The listing builds one solid part. Answer for the finished solid, in the listing's coordinates (mm). A direction names the side the tool comes from. Give positions to 0.01 mm unless a question says otherwise; leave off trailing zeros. Write each loop counter-clockwise with the first axis right and the second up, starting at its lowest first coordinate (ties: lowest second). Pieces come first, ordered by that corner, then holes. Notation, with made-up numbers: M 52.25,38 L 75.25,38 A18 cw 75.25,71 Z; hole C 12,-22.5 d9. An arc over 180 degrees is marked long. Answer as a JSON object with one key per item and string values.
```python
from build123d import *

# Parameters (mm, degrees)
SKETCH1_W               = 381
SKETCH1_H               = 76.2
BOSS_EXTRUDE1_DEPTH     = 14
SKETCH2_W               = 353.0000052
SKETCH2_H               = 48.2
CUT_EXTRUDE1_DEPTH      = 14
SKETCH5_W               = 381
SKETCH5_H               = 13.97
BOSS_EXTRUDE2_DEPTH     = 76.2
SKETCH6_W               = 353.0000052
SKETCH6_H               = 48.2
CUT_EXTRUDE2_DEPTH      = 76.2
SKETCH3_W               = 13.9999974
SKETCH3_H               = 14
BOSS_EXTRUDE3_DEPTH     = 429.26
SKETCH7_W               = 13.9999974
SKETCH7_H               = 101.6
CUT_EXTRUDE3_DEPTH      = 429.26
SKETCH10_W              = 13.9999974
SKETCH10_H              = 13.97
BOSS_EXTRUDE4_DEPTH     = 48.26
SKETCH11_W              = 353.0000052
SKETCH11_H              = 13.97
BOSS_EXTRUDE5_DEPTH     = 76.2
CUT_EXTRUDE4_DEPTH      = 352.863349754
CUT_EXTRUDE4_DEPTH_BACK = 352.863349754
SKETCH12_W              = 353.0000052
SKETCH12_H              = 48.2
SKETCH13_W              = 13.97
SKETCH13_H              = 13.97
BOSS_EXTRUDE6_DEPTH     = 48.26


with BuildPart() as part:
    # Sketch1 → Boss-Extrude1 (new body)
    with BuildSketch(Plane.XY):
        Rectangle(SKETCH1_W, SKETCH1_H)
    extrude(amount=BOSS_EXTRUDE1_DEPTH)

    # Sketch2 → Cut-Extrude1 (cut)
    with BuildSketch(Plane.XY.offset(14)):
        Rectangle(SKETCH2_W, SKETCH2_H)
    extrude(amount=-CUT_EXTRUDE1_DEPTH, mode=Mode.SUBTRACT)



with BuildPart() as body_2:
    # Sketch5 → Boss-Extrude2 (new body)
    with BuildSketch(Plane(origin=(0, -38.1, 0), x_dir=(1, 0, 0), z_dir=(0, 1, 0))):
        with Locations((0, -450.215)):
            Rectangle(SKETCH5_W, SKETCH5_H)
    extrude(amount=BOSS_EXTRUDE2_DEPTH)

    # Sketch6 → Cut-Extrude2 (cut)
    with BuildSketch(Plane(origin=(0, 0, 443.23), x_dir=(-1, 0, 0), z_dir=(0, 0, -1))):
        Rectangle(SKETCH6_W, SKETCH6_H)
    extrude(amount=-CUT_EXTRUDE2_DEPTH, mode=Mode.SUBTRACT)


with BuildPart() as part_1:
    add(part.part)

    add(body_2.part)  # Boss-Extrude3 merges body 2
    # Sketch3 → Boss-Extrude3 (add)
    with BuildSketch(Plane.XY.offset(14)):
        with Locations((-183.5000013, -31.1)):
            Rectangle(SKETCH3_W, SKETCH3_H)
        with Locations((-183.5000013, 31.1)):
            Rectangle(SKETCH3_W, SKETCH3_H)
        with Locations((183.5000013, -31.1)):
            Rectangle(SKETCH3_W, SKETCH3_H)
        with Locations((183.5000013, 31.1)):
            Rectangle(SKETCH3_W, SKETCH3_H)
    extrude(amount=BOSS_EXTRUDE3_DEPTH)

    # Sketch7 → Cut-Extrude3 (cut)
    with BuildSketch(Plane(origin=(0, 38.1, 0), x_dir=(1, 0, 0), z_dir=(0, 1, 0))):
        with Locations((183.5000013, -228.6)):
            Rectangle(SKETCH7_W, SKETCH7_H)
    extrude(amount=-CUT_EXTRUDE3_DEPTH, mode=Mode.SUBTRACT)

    # Sketch10 → Boss-Extrude4 (add)
    with BuildSketch(Plane(origin=(0, -24.1, 0), x_dir=(1, 0, 0), z_dir=(0, 1, 0))):
        with Locations((183.5000013, -170.815)):
            Rectangle(SKETCH10_W, SKETCH10_H)
        with Locations((183.5000013, -286.415)):
            Rectangle(SKETCH10_W, SKETCH10_H)
    extrude(amount=BOSS_EXTRUDE4_DEPTH)

    # Sketch11 → Boss-Extrude5 (add)
    with BuildSketch(Plane(origin=(0, -38.1, 0), x_dir=(1, 0, 0), z_dir=(0, 1, 0))):
        with Locations((0, -170.815)):
            Rectangle(SKETCH11_W, SKETCH11_H)
        with Locations((0, -286.415)):
            Rectangle(SKETCH11_W, SKETCH11_H)
    extrude(amount=BOSS_EXTRUDE5_DEPTH)

    # Sketch12 → Cut-Extrude4 (cut, two sides: drawn at the far end of the back side and taken through both)
    with BuildSketch(Plane(origin=(0, 0, 163.83), x_dir=(-1, 0, 0), z_dir=(0, 0, -1)).offset(-CUT_EXTRUDE4_DEPTH_BACK)):
        Rectangle(SKETCH12_W, SKETCH12_H)
    extrude(amount=CUT_EXTRUDE4_DEPTH + CUT_EXTRUDE4_DEPTH_BACK, mode=Mode.SUBTRACT)

    # Sketch13 → Boss-Extrude6 (add)
    with BuildSketch(Plane(origin=(0, -24.1, 0), x_dir=(1, 0, 0), z_dir=(0, 1, 0))):
        with Locations((132.6850026, -286.415)):
            Rectangle(SKETCH13_W, SKETCH13_H)
        with Locations((132.6850026, -170.815)):
            Rectangle(SKETCH13_W, SKETCH13_H)
    extrude(amount=BOSS_EXTRUDE6_DEPTH)


solid = part_1.part
```
1. A cutting plane is placed at C-C, the plane x = -34.5. Count the separate pieces of the cut face and the enclosed holes in it, plus the area to 3 significant figures.
Verdict:
{"separate pieces": "8", "enclosed holes": "0", "area": "1,570 mm2"}
2. For faces 4 (the flat face through (-176.5, -31, 367)), 5 (the flat face through (176.5, 0, 7)), 6 (the flat face through (183, 0, 293.4)), 7 (the flat face through (183, -31, 279.4)), determine the directions among +Z, -Z, +X, -X, +Y, -Y from which every point of the face is accessible in a straight line to the end or side of a thin tool.
Verdict:
{"face 4": "+Y, -Y", "face 5": "+Z, -Z", "face 6": "+X, -X", "face 7": "+X, +Y, -Y"}
3. A flat-ended cylindrical pin translates along its axis: pin 1 (15.5 mm diameter, centred on y = 28.5, z = 231, fed in from +X). Find the tip coordinate at first contact, or state that the pin passes through.
Verdict:
{"pin 1": "stops at x = -176.5"}
4. The mould has two halves that part along X. Classify faces 1 (the flat face through (183, 0, 279.43)), 2 (the flat face through (-2, -31, 443.23)), 3 (the flat face through (190.5, -26, 90)): released by +X, released by -X, zero draft, split by the parting line, or undercut.
Verdict:
{"face 1": "zero draft", "face 2": "undercut", "face 3": "released by +X"}
5. Consider line 1 along Z through (x, y) = (102.5, -26); line 2 along X through (y, z) = (25, 429); line 3 along X through (y, z) = (-28, 207). Determine where each line is inside the solid, lowest interval first.
Verdict:
{"line 1": "z = 0 to 14, 163.83 to 177.8, 279.43 to 293.4, 443.23 to 457.2", "line 2": "x = -190.5 to -176.5, 176.5 to 190.5", "line 3": "x = -190.5 to -176.5"}
6. A cutting plane is placed at A-A, the plane z = 421.5. Give the vertices of the cut face in (x, y).
Verdict:
{"outline": "M -190.5,-38.1 L -176.5,-38.1 L -176.5,-24.1 L -190.5,-24.1 Z; M -190.5,24.1 L -176.5,24.1 L -176.5,38.1 L -190.5,38.1 Z; M 176.5,-38.1 L 190.5,-38.1 L 190.5,-24.1 L 176.5,-24.1 Z; M 176.5,24.1 L 190.5,24.1 L 190.5,38.1 L 176.5,38.1 Z"}
7. A cutting plane is placed at B-B, the plane z = 270.5. Give the vertices of the cut face in (x, y), plus the area to 3 significant figures.
Verdict:
{"outline": "M -190.5,-38.1 L -176.5,-38.1 L -176.5,-24.1 L -190.5,-24.1 Z; M -190.5,24.1 L -176.5,24.1 L -176.5,38.1 L -190.5,38.1 Z", "area": "392 mm2"}
